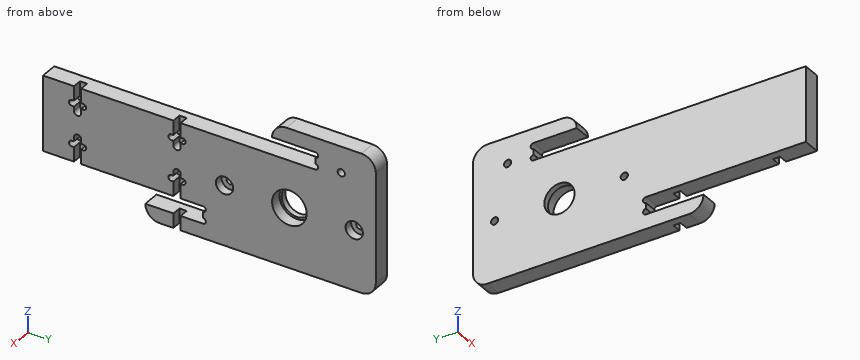
```python
from build123d import *

# Parameters (mm, degrees)
SKETCH1_W                          = 63
SKETCH1_H                          = 120
SKETCH1_R                          = 10.5
BOSS_EXTRUDE1_DEPTH                = 12
BOSS_EXTRUDE2_DEPTH                = 12
SKETCH9_W                          = 52
SKETCH9_H                          = 111
BOSS_EXTRUDE3_DEPTH                = 12
SKETCH11_W                         = 10
SKETCH11_H                         = 160
BOSS_EXTRUDE4_DEPTH                = 12
F_5_0_5_DIAMETER_HOLE1_D           = 5
LINEAR_RAIL_MOUNT_HOLE_D           = 5
LINEAR_RAIL_MOUNT_HOLE_CBORE_D     = 12
LINEAR_RAIL_MOUNT_HOLE_CBORE_DEPTH = 6
SKETCH27_R                         = 12
CUT_EXTRUDE1_DEPTH                 = 8
CUT_EXTRUDE2_REACH                 = 181.876
FILLET1_R                          = 10
CUT_EXTRUDE3_DEPTH                 = 8
CUT_EXTRUDE4_DEPTH                 = 6.5
LPATTERN1_COUNT                    = 2
LPATTERN1_PITCH                    = 69
MIRROR1_COPY_1_DEPTH               = 8
MIRROR1_COPY_2_DEPTH               = 6.5


with BuildPart() as part:
    # Sketch1 → Boss-Extrude1 (new body)
    with BuildSketch(Plane(origin=(0, 0, 0), x_dir=(0, 0, -1), z_dir=(1, 0, 0))):
        Rectangle(SKETCH1_W, SKETCH1_H)
        Circle(SKETCH1_R, mode=Mode.SUBTRACT)
    extrude(amount=BOSS_EXTRUDE1_DEPTH)

    # Sketch8 → Boss-Extrude2 (add)
    with BuildSketch(Plane.ZY):
        Polygon((44.5, 18), (44.5, -12), (54.5, -12), (54.5, 60), (31.5, 60), (31.5, -60), (32.5, -60), (32.5, 18), align=None)
    extrude(amount=-BOSS_EXTRUDE2_DEPTH)

    # Sketch9 → Boss-Extrude3 (add)
    with BuildSketch(Plane.ZY):
        with Locations((6.5, -115.5)):
            Rectangle(SKETCH9_W, SKETCH9_H)
    extrude(amount=-BOSS_EXTRUDE3_DEPTH)

    # Sketch11 → Boss-Extrude4 (add)
    with BuildSketch(Plane(origin=(12, 0, 0), x_dir=(0, 0, -1), z_dir=(1, 0, 0))):
        with Locations((36.5, -20)):
            Rectangle(SKETCH11_W, SKETCH11_H)
    extrude(amount=-BOSS_EXTRUDE4_DEPTH)

    # Ø5.0 (5) Diameter Hole1 (through all)
    with Locations(Plane(origin=(12, 0, 0), x_dir=(0, 0, -1), z_dir=(1, 0, 0))):
        with Locations((-36.5, 36)):
            Hole(F_5_0_5_DIAMETER_HOLE1_D / 2)

    # Linear Rail Mount Hole (through all)
    with Locations(Plane(origin=(12, 0, 0), x_dir=(0, 0, -1), z_dir=(1, 0, 0))):
        with Locations((0, -45), (0, 45)):
            CounterBoreHole(LINEAR_RAIL_MOUNT_HOLE_D / 2, LINEAR_RAIL_MOUNT_HOLE_CBORE_D / 2, LINEAR_RAIL_MOUNT_HOLE_CBORE_DEPTH)

    # Sketch27 → Cut-Extrude1 (cut)
    with BuildSketch(Plane(origin=(12, 0, 0), x_dir=(0, 0, -1), z_dir=(1, 0, 0))):
        Circle(SKETCH27_R)
    extrude(amount=-CUT_EXTRUDE1_DEPTH, mode=Mode.SUBTRACT)

    # Sketch28 → Cut-Extrude2 (cut, up to next)
    with BuildSketch(Plane(origin=(12, 0, 0), x_dir=(0, 0, -1), z_dir=(1, 0, 0)), mode=Mode.PRIVATE) as cut_extrude2_sk1:
        with BuildLine():
            Line((-44.5, 18), (-40.5, 18))
            ThreePointArc((-40.5, 18), (-42.5, 20), (-44.5, 18))
        make_face()
    cut_extrude2_tool1 = extrude(cut_extrude2_sk1.sketch, amount=-CUT_EXTRUDE2_REACH, mode=Mode.PRIVATE) & part.part
    # Sketch28 → Cut-Extrude2 (cut, up to next)
    with BuildSketch(Plane(origin=(12, 0, 0), x_dir=(0, 0, -1), z_dir=(1, 0, 0)), mode=Mode.PRIVATE) as cut_extrude2_sk2:
        with BuildLine():
            Line((-36.5, 18), (-32.5, 18))
            ThreePointArc((-32.5, 18), (-34.5, 20), (-36.5, 18))
        make_face()
    cut_extrude2_tool2 = extrude(cut_extrude2_sk2.sketch, amount=-CUT_EXTRUDE2_REACH, mode=Mode.PRIVATE) & part.part
    # Sketch28 → Cut-Extrude2 (cut, up to next)
    with BuildSketch(Plane(origin=(12, 0, 0), x_dir=(0, 0, -1), z_dir=(1, 0, 0)), mode=Mode.PRIVATE) as cut_extrude2_sk3:
        with BuildLine():
            Line((19.5, -60), (23.5, -60))
            ThreePointArc((23.5, -60), (21.5, -58), (19.5, -60))
        make_face()
    cut_extrude2_tool3 = extrude(cut_extrude2_sk3.sketch, amount=-CUT_EXTRUDE2_REACH, mode=Mode.PRIVATE) & part.part
    # Sketch28 → Cut-Extrude2 (cut, up to next)
    with BuildSketch(Plane(origin=(12, 0, 0), x_dir=(0, 0, -1), z_dir=(1, 0, 0)), mode=Mode.PRIVATE) as cut_extrude2_sk4:
        with BuildLine():
            Line((27.5, -60), (31.5, -60))
            ThreePointArc((31.5, -60), (29.5, -58), (27.5, -60))
        make_face()
    cut_extrude2_tool4 = extrude(cut_extrude2_sk4.sketch, amount=-CUT_EXTRUDE2_REACH, mode=Mode.PRIVATE) & part.part
    add(cut_extrude2_tool1.solids().sort_by_distance((12, 18.848826, 42.5))[0], mode=Mode.SUBTRACT)
    add(cut_extrude2_tool2.solids().sort_by_distance((12, 18.848826, 34.5))[0], mode=Mode.SUBTRACT)
    add(cut_extrude2_tool3.solids().sort_by_distance((12, -59.151174, -21.5))[0], mode=Mode.SUBTRACT)
    add(cut_extrude2_tool4.solids().sort_by_distance((12, -59.151174, -29.5))[0], mode=Mode.SUBTRACT)

    # Fillet1
    fillet1_edges = [part.edges().sort_by_distance(p)[0] for p in [
        (6, -12, 54.5),
        (6, -100, -41.5),
        (6, 60, 54.5),
        (6, 60, -41.5),
    ]]
    fillet(fillet1_edges, radius=FILLET1_R - 0.0001)  # a hair under: the kernel refuses the full size

    # Sketch29 → Cut-Extrude3 (cut)
    with BuildSketch(Plane(origin=(12, 0, 0), x_dir=(0, 0, -1), z_dir=(1, 0, 0))):
        with BuildLine():
            Line((9.5, -143), (9.5, -151))
            ThreePointArc((9.5, -151), (7.5, -153), (5.5, -151))
            Line((5.5, -151), (5.5, -143))
            ThreePointArc((5.5, -143), (7.5, -141), (9.5, -143))
        make_face()
    cut_extrude3 = extrude(amount=-CUT_EXTRUDE3_DEPTH, mode=Mode.SUBTRACT)

    # Sketch31 → Cut-Extrude4 (cut)
    with BuildSketch(Plane(origin=(12, 0, 0), x_dir=(0, 0, -1), z_dir=(1, 0, 0))):
        with BuildLine():
            Line((65.397486198, -149.5), (2.5, -149.5))
            ThreePointArc((2.5, -149.5), (0, -147), (2.5, -144.5))
            Line((2.5, -144.5), (65.397486198, -144.5))
            ThreePointArc((65.397486198, -144.5), (67.897486198, -147), (65.397486198, -149.5))
        make_face()
    cut_extrude4 = extrude(amount=-CUT_EXTRUDE4_DEPTH, mode=Mode.SUBTRACT)

    # LPattern1: Cut-Extrude3, Cut-Extrude4 ×2
    with Locations(*[(0, i * LPATTERN1_PITCH, 0) for i in range(1, LPATTERN1_COUNT)]):
        add(cut_extrude3, mode=Mode.SUBTRACT)
        add(cut_extrude4, mode=Mode.SUBTRACT)

    # Mirror1: Cut-Extrude3, Cut-Extrude4 across plane
    add(cut_extrude3.mirror(Plane(origin=(0, 0, 6.5), x_dir=(1, 0, 0), z_dir=(0, 0, -1))), mode=Mode.SUBTRACT)
    add(cut_extrude4.mirror(Plane(origin=(0, 0, 6.5), x_dir=(1, 0, 0), z_dir=(0, 0, -1))), mode=Mode.SUBTRACT)

    # Mirror1 copy 1 sketch → Mirror1 copy 1 (cut)
    with BuildSketch(Plane(origin=(12, 69, 13), x_dir=(0, 0, 1), z_dir=(1, 0, 0))):
        with BuildLine():
            Line((9.5, 143), (9.5, 151))
            ThreePointArc((9.5, 151), (7.5, 153), (5.5, 151))
            Line((5.5, 151), (5.5, 143))
            ThreePointArc((5.5, 143), (7.5, 141), (9.5, 143))
        make_face()
    extrude(amount=-MIRROR1_COPY_1_DEPTH, mode=Mode.SUBTRACT)

    # Mirror1 copy 2 sketch → Mirror1 copy 2 (cut)
    with BuildSketch(Plane(origin=(12, 69, 13), x_dir=(0, 0, 1), z_dir=(1, 0, 0))):
        with BuildLine():
            Line((65.397486198, 149.5), (2.5, 149.5))
            ThreePointArc((2.5, 149.5), (0, 147), (2.5, 144.5))
            Line((2.5, 144.5), (65.397486198, 144.5))
            ThreePointArc((65.397486198, 144.5), (67.897486198, 147), (65.397486198, 149.5))
        make_face()
    extrude(amount=-MIRROR1_COPY_2_DEPTH, mode=Mode.SUBTRACT)


solid = part.part
```
Geometry check sheet. Reference: the model listing, model coordinates, mm. Coordinates: 2 decimals unless noted, no trailing zeros. Write each loop counter-clockwise with the first axis right and the second up, starting at its lowest first coordinate (ties: lowest second). Pieces come first, ordered by that corner, then holes. Notation, with made-up numbers: M 71.25,-30 L 105.25,-30 A6 cw 105.25,-22 Z; hole C 74.25,30 d5. An arc over 180 degrees is marked long. Use one line per item in the form item = value. Start each with the question number.
1) Section check C-C on z = -14.5. Enter the section's corners in (x, y), and give its area (3 significant figures).
2) Section check D-D on y = -35.5. Enter the section's corners in (x, z), and give its area (3 significant figures).
3) Thickness scan on probe 1 along Z at (x, y) = (2.85, 0); probe 2 along Y at (x, z) = (5, 1); probe 3 along Y at (x, z) = (4.5, 1.5). Record the ranges inside material, lowest first. Write a range as from..to.
4) Section check B-B on x = 2. State how many separate pieces and enclosed holes the cut face has, and give its area (3 significant figures).
5) Go/stop test with flat-tipped pins: pin 1 Ø3 at (y, z) = (-78.5, 21.5) entering from +X; pin 2 Ø1.5 at (y, z) = (-145.5, 25.5) entering from -X; pin 3 Ø3 at (y, z) = (-81, -7.5) entering from +X; pin 4 Ø2.5 at (x, y) = (9, -148.5) entering from -Z. Record where each tip stops, or that it passes through.
6) Section check A-A on y = -65.5. Enter the section's corners in (x, z).
Responses:
q1.outline = M 0,-171 L 12,-171 L 12,-149.5 L 5.5,-149.5 L 5.5,-144.5 L 12,-144.5 L 12,-80.5 L 5.5,-80.5 L 5.5,-75.5 L 12,-75.5 L 12,60 L 0,60 Z
q1.area = 2,710 mm2
q2.outline = M 0,-41.5 L 12,-41.5 L 12,32.5 L 0,32.5 Z
q2.area = 888 mm2
q3.probe_1 = -41.5..-10.5, 10.5..32.5, 44.5..54.5
q3.probe_2 = -171..-47.29, -42.71..-11.96, 11.96..42.71, 47.29..60
q3.probe_3 = -171..-47, -43..-11.91, 11.91..43, 47..60
q4.separate_pieces = 1
q4.enclosed_holes = 4
q4.area = 15,800 mm2
q5.pin_1 = 5.5
q5.pin_2 = 0
q5.pin_3 = 4
q5.pin_4 = -19.5
q6.outline = M 0,-41.5 L 12,-41.5 L 12,-31.5 L 0,-31.5 Z; M 0,-19.5 L 12,-19.5 L 12,32.5 L 0,32.5 Z
